Autodesk Inventor part; units mm, degrees
ref_plane "SideProfilePlane" through (0, 12, 0) normal (0, 1, 0) x (-1, 0, 0)
ref_plane "HeadMountPlane" through (29, 0, 3) normal (0, 0, 1) x (1, 0, 0)
ref_plane "YZ Plane" through (0, 0, 0) normal (1, 0, 0) x (0, 1, 0)
sketch "Body" plane through (0, 0, 0) normal (0, 0, 1) x (1, 0, 0)
  circle A0 centre (0, 0) radius 10
  line L0 (0, 0) -> (29, 0) construction
  circle A1 centre (29, 0) radius 7.75
  line L1 (0.7759, 9.9699) -> (29.6013, 7.7266)
  line L2 (0.7759, -9.9699) -> (29.6013, -7.7266)
  dimension "SmallDiameter" = 20
  dimension "d1" = 29
  dimension "LargeDiameter" = 15.5
extrude "BodyFeature" add sketch "Body" along normal blind 18
ref_plane "SideProfilePlane" through (0, 12, 0) normal (0, 1, 0) x (-1, 0, 0)
sketch "SideProfile" plane through (0, 12, 0) normal (0, 1, 0) x (-1, 0, 0)
  line L0 (10, 18) -> (-0.7759, 18) construction
  line L1 (10, 18) -> (10, 15)
  line L2 (10, 15) -> (-6, 15)
  line L3 (-6, 15) -> (-20.75, 0)
  line L4 (-20.75, 0) -> (-36.75, 0)
  line L5 (-29.6013, 0) -> (-0.7759, 0) construction
  line L6 (-36.75, 0) -> (-36.75, 18) construction
  line L7 (-29.6013, 18) -> (-36.75, 18) construction
  line L8 (-29.6013, 18) -> (-0.7759, 18) construction
  line L9 (-22.0074, 3) -> (-7.2574, 18)
  line L10 (-36.75, 3) -> (-22.0074, 3)
  line L11 (-36.75, 0) -> (-36.75, 3)
  line L12 (10, 18) -> (-7.2574, 18)
  dimension "Thickness" = 3
  dimension "d15" = 3
  dimension "d16" = 3
  dimension "d17" = 16
  dimension "d18" = 16
extrude "SideProfileFeature" cut sketch "SideProfile" against normal through all keep common part
fillet "BodyFilletsFeate" radius 3 3 edges at (6, 0, 15) (22.0074, 0, 3) (7.2574, 0, 18)
ref_plane "HeadMountPlane" through (29, 0, 3) normal (0, 0, 1) x (1, 0, 0)
sketch "HeadMountHole" plane through (29, 0, 3) normal (0, 0, 1) x (1, 0, 0)
  circle A0 centre (-2, 0) radius 3.25
  arc A1 (0.6013, -7.7266) -> (0.6013, 7.7266) centre (0, 0) ccw construction
  line L0 (-2, 0) -> (0, 0) construction
  point P0 (-29, 0)
  dimension "d307" = 2
  dimension "d308" = 6.5
hole "HeadMountHoleFeature" at (27, 0, 3) direction (0, 0, -1) diameter 5 end through all
sketch "BodyMountHole" plane through (0, 0, 18) normal (0, 0, 1) x (1, 0, 0)
  arc A0 (0.7759, 9.9699) -> (0.7759, -9.9699) centre (0, 0) ccw
hole "BodyMountHoleFeature" at (0, 0, 18) direction (0, 0, -1) diameter 6 end through all
fillet "BodyFillets2Feature" radius 4 1 edges at (20.75, 0, 0)
equation "\"d16\" = Thickness"
properties part number "ShoulderConnectorBodyFinal"
Here's how the part is built. I have some questions about the finished solid (model axes, mm). A direction names the side the tool comes from. Give positions to 0.01 mm unless a question says otherwise; leave off trailing zeros. Write each loop counter-clockwise with the first axis right and the second up, starting at its lowest first coordinate (ties: lowest second). Pieces come first, ordered by that corner, then holes. Notation, with made-up numbers: (-7.75, -17) -> (5.25, -17) arc R35 cw to (5.25, 20) -> close; hole circle Ø1 at (57.25, 14.5). An arc over 180 degrees is marked (long way). Use one line per item in the form item = value. Start each with the question number.
1. Imagine slicing it at A-A on y = 0. List the corners of the cut face in (x, z) for me.
2. Imagine slicing it at B-B on x = 0. List the corners of the cut face in (y, z) for me.
3. If I drill on L1, parallel to Z at x = 30.5, y = -1.5; L2, parallel to Z at x = -3, y = 8.25; L3, parallel to X at y = 0, z = 16.05, over which ranges is the centre line in solid material (lowest first)?
4. On a 3-axis mill with a long thin cutter (end or side, diameter ignored), from which of +Z, -Z, +X, -X, +Y, -Y can I reach the whole of each face in a straight line? I mean faces 4 (the face through (15.121, 8.853, 8.291)), 5 (the face through (30, 0, 3)), 6 (the face through (-3, -2, 15)). Say none if no direction works.
5. Imagine slicing it at D-D on y = 6.5. List the corners of the cut face in (x, z) for me, plus the area to 3 significant figures.
6. Thinking about a two-plate mould opening in X: for faces 1 (the face through (24.52, 0.33, 1.48)), 2 (the face through (15.121, -8.853, 8.291)), 3 (the face through (29, -2, 0)), which applies, +X half, -X half, draft (parallel to the pull), parting line (faces both ways), or undercut?
7. Will these pins go through, and if not, where does the flat tip stop? pin 1 Ø8 at (y, z) = (-1, 11.5) entering from -X; pin 2 Ø3 at (x, z) = (1.5, 14) entering from -Y; pin 3 Ø7.5 at (x, y) = (-5.5, 2) entering from -Z; pin 4 Ø4 at (x, y) = (27, 0) entering from -Z.
8. Imagine slicing it at C-C on y = 2. List the corners of the cut face in (x, z) for me.
Entries:
q1.outline = (-10, 15) -> (-3, 15) -> (-3, 18) -> (-10, 18) -> close; (3, 15) -> (4.74, 15) arc R3 cw to (6.88, 14.1) -> (19.57, 1.2) arc R4 ccw to (22.43, 0) -> (24.5, 0) -> (24.5, 3) -> (23.26, 3) arc R3 cw to (21.13, 3.9) -> (8.14, 17.1) arc R3 ccw to (6, 18) -> (3, 18) -> close; (29.5, 0) -> (36.75, 0) -> (36.75, 3) -> (29.5, 3) -> close
q2.outline = (-10, 15) -> (-3, 15) -> (-3, 18) -> (-10, 18) -> close; (3, 15) -> (10, 15) -> (10, 18) -> (3, 18) -> close
q3.L1 = 0 to 3
q3.L2 = 15 to 18
q3.L3 = -10 to -3, 3 to 9.17
q4.face_4 = +Z, -Z, +X, +Y
q4.face_5 = +Z, +X, +Y, -Y
q4.face_6 = -Z, -X, +Y, -Y
q5.outline = (-7.6, 15) -> (4.74, 15) arc R3 cw to (6.88, 14.1) -> (19.57, 1.2) arc R4 ccw to (22.43, 0) -> (33.22, 0) -> (33.22, 3) -> (23.26, 3) arc R3 cw to (21.13, 3.9) -> (8.14, 17.1) arc R3 ccw to (6, 18) -> (-7.6, 18) -> close
q5.area = 141 mm²
q6.face_1 = undercut
q6.face_2 = +X half
q6.face_3 = draft
q7.pin_1 = -10
q7.pin_2 = -9.99
q7.pin_3 = 15
q7.pin_4 = through
q8.outline = (-9.8, 15) -> (-2.24, 15) -> (-2.24, 18) -> (-9.8, 18) -> close; (2.24, 15) -> (4.74, 15) arc R3 cw to (6.88, 14.1) -> (19.57, 1.2) arc R4 ccw to (22.43, 0) -> (25.5, 0) -> (25.5, 3) -> (23.26, 3) arc R3 cw to (21.13, 3.9) -> (8.14, 17.1) arc R3 ccw to (6, 18) -> (2.24, 18) -> close; (28.5, 0) -> (36.49, 0) -> (36.49, 3) -> (28.5, 3) -> close
